from build123d import *

# Parameters (mm, degrees)
F0_R     = 1.5
F1_DEPTH = 2.5
F3_DEPTH = 15
F4_R     = 5


with BuildPart() as f1:
    # F0 (on Front) → F1 (new body)
    with BuildSketch(Plane.XZ):
        with Locations((57.5, 2.5)):
            Circle(F0_R)
        with BuildLine():
            ThreePointArc((4, 2.5), (2.5, 4), (1, 2.5))
            ThreePointArc((1, 2.5), (2.5, 1), (4, 2.5))
        make_face()
        Polygon((0, 2.5), (0, 0), (60, 0), (60, 2.5), (60, 5), (0, 5), align=None)
        with BuildLine():
            ThreePointArc((4, 2.5), (2.5, 1), (1, 2.5))
            ThreePointArc((1, 2.5), (2.5, 4), (4, 2.5))
        make_face(mode=Mode.SUBTRACT)
        with Locations((57.5, 2.5)):
            Circle(F0_R, mode=Mode.SUBTRACT)
    extrude(amount=F1_DEPTH)

    # F2 (on face) → F3 (join)
    with BuildSketch(Plane.XZ.offset(2.5)):
        Polygon((50, 5), (30, 5), (10, 5), (10, 0), (50, 0), align=None)
    extrude(amount=F3_DEPTH)

    # F4
    f4_edges = [f1.edges().sort_by_distance(p)[0] for p in [
        (10, -17.5, 2.5),
        (50, -17.5, 2.5),
    ]]
    fillet(f4_edges, radius=F4_R)


solid = f1.part
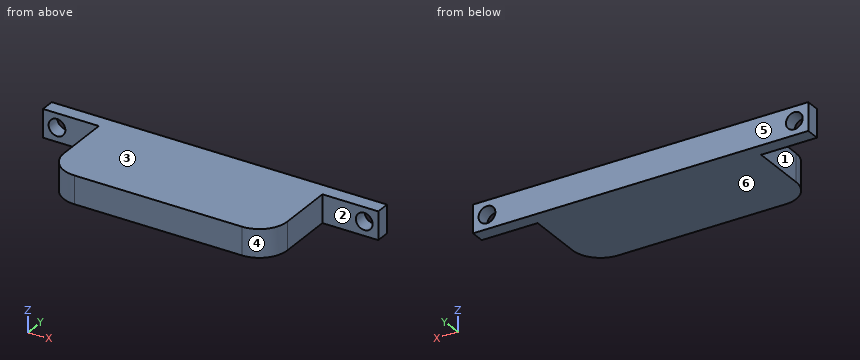
CAD build for the part. Positions are in the model's coordinates, mm. Face numbers are marked on the shaded views. A direction names the side the tool comes from. Round coordinates to 2 decimals unless told otherwise and drop trailing zeros. Order: outer loops, then holes, each group sorted by start corner. A loop starts at its lowest first (then second) coordinate and runs counter-clockwise, first axis right, second up. Notation, with made-up numbers: (52.5, 57) -> (82.5, 57) arc R8 cw to (82.5, 65) -> close; hole circle Ø10 at (37, 7.5). An arc over 180 degrees is marked (long way). Write item = value, one per line. Start each with the question number.
(1) Pin check, flat tips, straight feed: P1, Ø1.5, axis at x = 5, z = 3, coming from the -Y side; P2, Ø2.5, axis at x = 2.5, z = 2.5, coming from the +Y side; P3, Ø1.5, axis at y = -6.5, z = 3.5, coming from the -X side; P4, Ø2, axis at x = 47.5, z = 3, coming from the -Y side. Stop position of each tip, or through.
(2) Which spindle directions (+Z, -Z, +X, -X, +Y, -Y) get a long thin tool onto all of the face, cutting with end or side? Do the marked faces 1, 2 and 3. Say none if no direction does.
(3) Cut at A-A, the plane z = 3.4. List the corners of the cut face in (x, y).
(4) Cut at B-B, the plane x = 2.5. List the corners of the cut face in (y, z).
(5) Pull direction Y, two halves, no side cores. Call the marked faces 4, 5 and 6: released by +Y, released by -Y, zero draft, split by the parting line, or undercut.
(6) Cut at D-D, the plane y = -14.5. List the corners of the cut face in (x, z).
(7) Probe line 1 (Z direction, x = 2.5, y = -1.4); line 2 (Y direction, x = 54.5, z = 0.65); line 3 (X direction, y = -7, z = 4.3). List the from-to ranges inside material, lowest first. Write a range as [from, to].
(8) Cut at C-C, the plane y = -5. List the corners of the cut face in (x, z).
Model answer:
q1.P1 = -2.5
q1.P2 = through
q1.P3 = 10
q1.P4 = -17.27
q2.face_1 = +Z, -Z, -X, -Y
q2.face_2 = +Z, -Z, +X, -Y
q2.face_3 = +Z, +X, -X, +Y, -Y
q3.outline = (0, -2.5) -> (1.3, -2.5) -> (1.3, 0) -> (0, 0) -> close; (3.7, -2.5) -> (10, -2.5) -> (10, -12.5) arc R5 ccw to (15, -17.5) -> (45, -17.5) arc R5 ccw to (50, -12.5) -> (50, -2.5) -> (56.3, -2.5) -> (56.3, 0) -> (3.7, 0) -> close; (58.7, -2.5) -> (60, -2.5) -> (60, 0) -> (58.7, 0) -> close
q4.outline = (-2.5, 0) -> (0, 0) -> (0, 1) -> (-2.5, 1) -> close; (-2.5, 4) -> (0, 4) -> (0, 5) -> (-2.5, 5) -> close
q5.face_4 = released by -Y
q5.face_5 = released by +Y
q5.face_6 = zero draft
q6.outline = (10.42, 0) -> (49.58, 0) -> (49.58, 5) -> (10.42, 5) -> close
q7.line_1 = [0, 1], [4, 5]
q7.line_2 = [-2.5, 0]
q7.line_3 = [10, 50]
q8.outline = (10, 0) -> (50, 0) -> (50, 5) -> (10, 5) -> close
